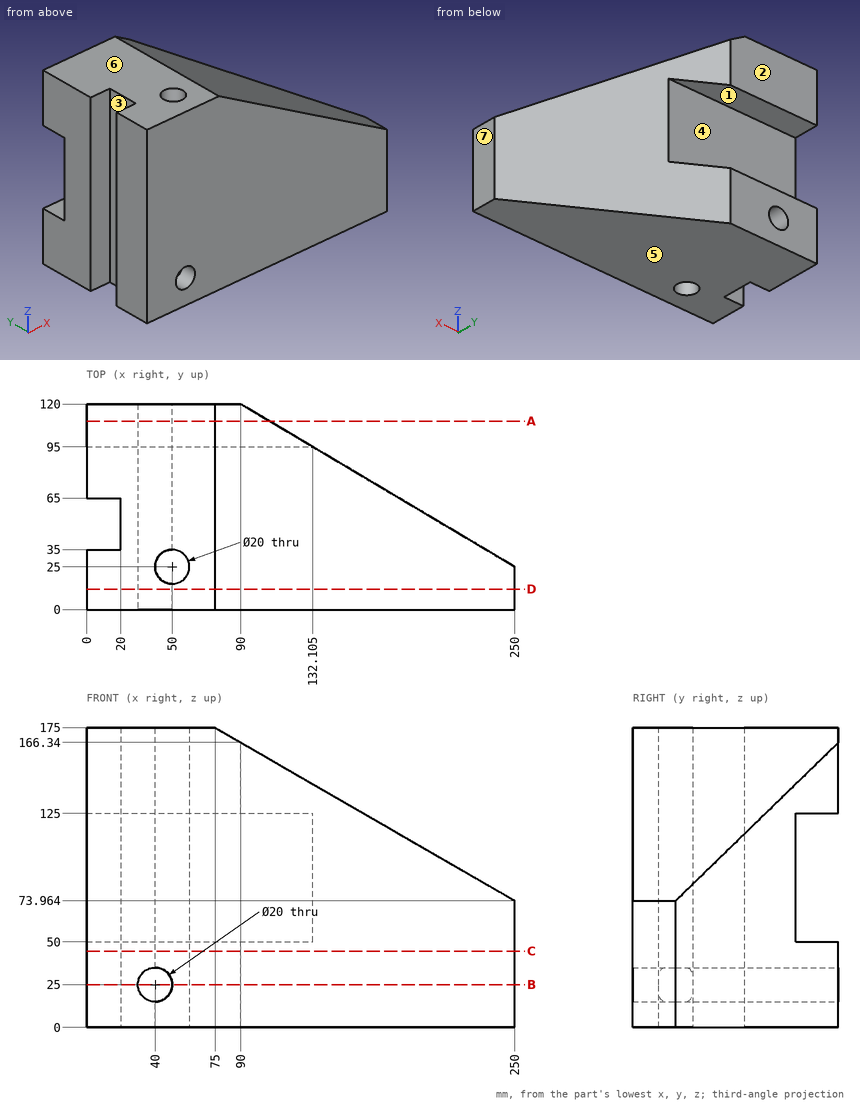
For this review, use the dimensioned drawing (mm, ordinates from the lowest corner) and the shaded views. A direction names the side the tool comes from. Give positions to 0.01 mm unless a question says otherwise; leave off trailing zeros. Order: outer loops, then holes, each group sorted by start corner. A loop starts at its lowest first (then second) coordinate and runs counter-clockwise, first axis right, second up. Notation, with made-up numbers: (-5, 33.25) - (44, 33.25) arc R28 cw to (44, 66.25) - close; hole circle Ø2 at (29.25, 4). An arc over 180 degrees is marked (long way). Use a Markdown table: item, result. Add a question column.
(1) Add section A-A on y = 110. Give the boundary of the cut face in (x, z).
(2) Clearance check with flat-ended pins moving along their axes: P1, Ø4, axis at y = 24.5, z = 146.5, coming from the +X side; P2, Ø4, axis at y = 52.5, z = 52.5, coming from the -X side; P3, Ø5, axis at x = 197.5, z = 90.5, coming from the +Y side. State where each tip first meets the part, or that it passes through.
(3) Mouldability with a two-part tool opening along Z and no side actions: class the marked faces 4, 5, 6 and 7 as +Z half, -Z half, draft (parallel to the pull), parting line (faces both ways), or undercut.
(4) Add section B-B on z = 25. Give the boundary of the cut face in (x, y), then the cut area to 3 significant figures.
(5) Add section C-C on z = 44.5. Give the boundary of the cut face in (x, y).
(6) Wall thickness on probe 1 along Z at (x, y) = (40, 102); probe 2 along Y at (x, z) = (50, 128); probe 3 along Y at (x, z) = (50, 71): over which ranges is each line inside the solid? List them lowest first. Write a range as [from, to].
(7) Add section D-D on y = 12. Give the boundary of the cut face in (x, z), then the cut area to 3 significant figures.
(8) Machinability: for the marked faces 1, 2 and 3, which of the approach directions +Z, -Z, +X, -X, +Y, -Y give a long, thin tool a straight path to every point of the face, cutting with its end or side? Answer none if there is none.
Report:
| question | item | result |
|---|---|---|
| 1 | outline | (0, 0) - (106.84, 0) - (106.84, 50) - (0, 50) - close; (0, 125) - (106.84, 125) - (106.84, 156.62) - (75, 175) - (0, 175) - close; hole circle Ø20 at (40, 25) |
| 2 | P1 | stops at x = 127.83 |
| 2 | P2 | stops at x = 20 |
| 2 | P3 | stops at y = 57.66 |
| 3 | face 4 | undercut |
| 3 | face 5 | -Z half |
| 3 | face 6 | +Z half |
| 3 | face 7 | draft |
| 4 | outline | (0, 0) - (30, 0) - (30, 120) - (0, 120) - (0, 65) - (20, 65) - (20, 35) - (0, 35) - close; (50, 0) - (250, 0) - (250, 25) - (90, 120) - (50, 120) - (50, 35) arc R10 cw to (50, 15) - close |
| 4 | area | 19,200 mm² |
| 5 | outline | (0, 0) - (250, 0) - (250, 25) - (90, 120) - (0, 120) - (0, 65) - (20, 65) - (20, 35) - (0, 35) - close; hole circle Ø20 at (50, 25) |
| 6 | probe 1 | z = [0, 15], [35, 50], [125, 175] |
| 6 | probe 2 | y = [0, 15], [35, 120] |
| 6 | probe 3 | y = [0, 15], [35, 95] |
| 7 | outline | (0, 0) - (250, 0) - (250, 73.96) - (75, 175) - (0, 175) - close; hole circle Ø20 at (40, 25) |
| 7 | area | 34,600 mm² |
| 8 | face 1 | +X, -X, +Y |
| 8 | face 2 | +Z, -Z, +X, -X, +Y |
| 8 | face 3 | +Z, -Z, -X |
